Verification items for the finished model (mm, model axes). Face numbers are marked on the shaded views. A direction names the side the tool comes from. Round coordinates to 2 decimals unless told otherwise and drop trailing zeros. Loops run counter-clockwise (first coordinate to the right, second up) from the corner with the lowest first, then second, coordinate; pieces in that order, holes last. Notation, with made-up numbers: M -38,33.25 L -17,33.25 A13 cw -17,37.25 Z; hole C 9.5,21.5 d10. An arc over 180 degrees is marked long. One line per item, written item: value.
from build123d import *

# Parameters (mm, degrees)
SKETCH_1_W          = 100
SKETCH_1_H          = 40
EXTRUDE_1_DEPTH     = 19
SKETCH_2_R          = 9.811124868
EXTRUDE_2_DEPTH     = 14
SKETCH_3_W          = 13
SKETCH_3_H          = 13
CUT_EXTRUDE_1_DEPTH = 6
SKETCH_4_R          = 3
CUT_EXTRUDE_2_DEPTH = 110.544511501
SKETCH_5_R          = 3.5
CUT_EXTRUDE_3_DEPTH = 113.645461515
SKETCH_6_R          = 3.5
CUT_EXTRUDE_4_DEPTH = 110.366356801
SKETCH_7_W          = 87
SKETCH_7_H          = 13
CUT_EXTRUDE_6_DEPTH = 31
SKETCH_8_R          = 3.5
CUT_EXTRUDE_7_DEPTH = 109.710625056


with BuildPart() as part:
    # Эскиз1 → Бобышка-Вытянуть1 (new body)
    with BuildSketch(Plane(origin=(0, 0, 0), x_dir=(1, 0, 0), z_dir=(0, 1, 0))):
        with Locations((-50, 20)):
            Rectangle(SKETCH_1_W, SKETCH_1_H)
    extrude(amount=EXTRUDE_1_DEPTH)

    # Эскиз2 → Бобышка-Вытянуть2 (add)
    with BuildSketch(Plane(origin=(0, 19, 0), x_dir=(1, 0, 0), z_dir=(0, 1, 0))):
        with Locations(Location((-50, 20, 0), (0, 0, 270))):
            Circle(SKETCH_2_R)
    extrude(amount=EXTRUDE_2_DEPTH)

    # Эскиз3 → Вырез-Вытянуть1 (cut)
    with BuildSketch(Plane(origin=(0, 19, 0), x_dir=(1, 0, 0), z_dir=(0, 1, 0))):
        with Locations((-93.5, 6.5)):
            Rectangle(SKETCH_3_W, SKETCH_3_H)
    extrude(amount=-CUT_EXTRUDE_1_DEPTH, mode=Mode.SUBTRACT)

    # Эскиз4 → Вырез-Вытянуть2 (cut, through all)
    with BuildSketch(Plane(origin=(0, 13, 0), x_dir=(1, 0, 0), z_dir=(0, 1, 0))):
        with Locations(Location((-93.5, 6.5, 0), (0, 0, 270))):
            Circle(SKETCH_4_R)
    extrude(amount=-CUT_EXTRUDE_2_DEPTH, mode=Mode.SUBTRACT)

    # Эскиз5 → Вырез-Вытянуть3 (cut, through all)
    with BuildSketch(Plane(origin=(0, 33, 0), x_dir=(1, 0, 0), z_dir=(0, 1, 0))):
        with Locations(Location((-50, 20, 0), (0, 0, 270))):
            Circle(SKETCH_5_R)
    extrude(amount=-CUT_EXTRUDE_3_DEPTH, mode=Mode.SUBTRACT)

    # Эскиз6 → Вырез-Вытянуть4 (cut, through all)
    with BuildSketch(Plane(origin=(0, 19, 0), x_dir=(1, 0, 0), z_dir=(0, 1, 0))):
        with Locations(Location((-15.91089824, 20, 0), (0, 0, 270))):
            Circle(SKETCH_6_R)
    extrude(amount=-CUT_EXTRUDE_4_DEPTH, mode=Mode.SUBTRACT)

    # Эскиз7 → Вырез-Вытянуть6 (cut)
    with BuildSketch(Plane(origin=(0, 19, 0), x_dir=(1, 0, 0), z_dir=(0, 1, 0))):
        with Locations((-43.5, 6.5)):
            Rectangle(SKETCH_7_W, SKETCH_7_H)
    extrude(amount=CUT_EXTRUDE_6_DEPTH, mode=Mode.SUBTRACT)

    # Эскиз8 → Вырез-Вытянуть7 (cut, through all)
    with BuildSketch(Plane.XY.offset(-13)):
        with Locations((-50, 26)):
            Circle(SKETCH_8_R)
    extrude(amount=-CUT_EXTRUDE_7_DEPTH, mode=Mode.SUBTRACT)


solid = part.part
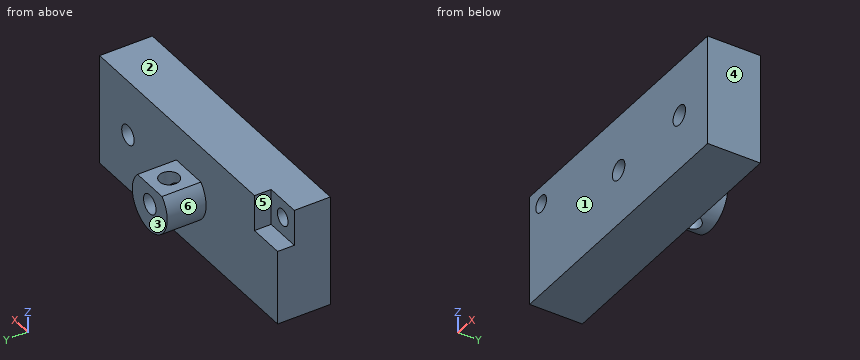
(1) Sectioned sample at B-B on x = -93.5. Enter the section's corners in (y, z), and give its area (3 significant figures).
Completed:
outline: M 0,-40 L 19,-40 L 19,-13 L 13,-13 L 13,-9.5 L 0,-9.5 Z; M 0,-3.5 L 13,-3.5 L 13,0 L 0,0 Z
area: 604 mm^2
(2) Mould release check, pull along Y, two halves, no side actions. Record for the marked faces 1, 2 and 3: +Y half, -Y half, draft (parallel to the pull), parting line (faces both ways), or undercut.
Completed:
face 1: -Y half
face 2: draft
face 3: +Y half
(3) Depth check by flat-ended pin: pin 1 Ø5.5 at (x, z) = (-50, -20) entering from -Y; pin 2 Ø9 at (x, y) = (-50, 26) entering from +Z; pin 3 Ø1.8 at (y, z) = (15, -9) entering from -X; pin 4 Ø4 at (x, z) = (-87.5, -10) entering from +Y. Enter the tip coordinate at first touch or a pass-through.
Completed:
pin 1: passes through
pin 2: stops at z = -13
pin 3: stops at x = -87
pin 4: stops at y = 19
(4) Sectioned sample at C-C on y = 21.5. Enter the section's corners in (x, z), and give its area (3 significant figures).
Completed:
outline: M -56.87,-13 A9.81 ccw long -43.13,-13 Z; hole C -50,-20 d7
area: 237 mm^2
(5) Tool access check on the marked faces 4, 5 and 6. Record the directions out of +Z, -Z, +X, -X, +Y, -Y that give a thin tool (end or side, any length) a straight path to the whole face; none if there is none.
Completed:
face 4: +Z, -Z, +X, +Y, -Y
face 5: +Z, -X, +Y
face 6: +Y
(6) Sectioned sample at D-D on z = -26. Enter the section's corners in (x, y).
Completed:
outline: M -100,0 L 0,0 L 0,19 L -42.24,19 L -42.24,33 L -57.76,33 L -57.76,19 L -100,19 Z; hole C -50,26 d7
(7) Thickness scan on L1, parallel to X at y = 16, z = -20; L2, parallel to Z at x = -50, y = 18.5; L3, parallel to X at y = 30, z = -20. Record the ranges inside material, lowest first. Write a range as from..to.
Completed:
L1: x = -100..-53.5, -46.5..-19.41, -12.41..0
L2: z = -40..-23.5, -16.5..0
L3: x = -59.81..-53.5, -46.5..-40.19
(8) Sectioned sample at A-A on z = -6.5. Enter the section's corners in (x, y), and give its area (3 significant figures).
Completed:
outline: M -100,0 L -96.5,0 L -96.5,13 L -100,13 Z; M -90.5,0 L 0,0 L 0,19 L -87,19 L -87,13 L -90.5,13 Z
area: 1,740 mm^2
